Part model, mm, in its own coordinate system. Give positions to 0.01 mm unless a question says otherwise; leave off trailing zeros. Order: outer loops, then holes, each group sorted by start corner. A loop starts at its lowest first (then second) coordinate and runs counter-clockwise, first axis right, second up. Notation, with made-up numbers: (54.5, 38.25) -> (113.5, 38.25) arc R7 cw to (113.5, 49.25) -> close; hole circle Ø2 at (-16.5, 8). An arc over 180 degrees is marked (long way). Write item = value, one per line. Start each with the question number.
(1) Probe line 1 along X through (y, z) = (7.75, 940.5); line 2 along Z through (x, y) = (-110.5, 10.75); line 3 along X through (y, z) = (1.5, 679). List the from-to ranges inside material, lowest first. Write a range as from..to.
(2) Saw through at B-B, the plane y = 10. List the corners of the cut face in (x, z).
(3) Flat gauge pins, fed straight in: pin 1 (10.5 mm diameter, centred on y = 9.5, z = 1421, fed in from +X); pin 2 (8 mm diameter, centred on y = 8.5, z = 2045, fed in from +X); pin 3 (5 mm diameter, centred on x = -36.5, y = 9.5, fed in from -Z). Where does each tip first touch, or does it go through?
(4) Saw through at A-A, the plane z = 985.5. List the corners of the cut face in (x, y).
from build123d import *

# Parameters (mm, degrees)
F0_W     = 266.7
F0_H     = 9.525
F1_DEPTH = 2286
F2_DEPTH = 25.4
F3_W     = 266.7
F3_H     = 9.525
F4_DEPTH = 25.4


with BuildPart() as f1:
    # F0 (on Top) → F1 (new body)
    with BuildSketch(Plane.XY):
        with Locations((11.780921, 11.16089)):
            Rectangle(F0_W, F0_H)
        Polygon((-131.094079, 6.39839), (-140.619079, -3.12661), (164.180921, -3.12661), (154.655921, 6.39839), (145.130921, 6.39839), (-121.569079, 6.39839), align=None)
    extrude(amount=F1_DEPTH)

    # F0 (on Top) → F2 (cut)
    with BuildSketch(Plane.XY):
        with Locations((11.780921, 11.16089)):
            Rectangle(F0_W, F0_H)
    extrude(amount=F2_DEPTH, mode=Mode.SUBTRACT)

    # F3 (on face) → F4 (cut)
    with BuildSketch(Plane.XY.offset(2286)):
        with Locations((11.780921, 11.16089)):
            Rectangle(F3_W, F3_H)
    extrude(amount=-F4_DEPTH, mode=Mode.SUBTRACT)


solid = f1.part
Results list:
q1.line_1 = -121.57..145.13
q1.line_2 = 25.4..2260.6
q1.line_3 = -135.99..159.55
q2.outline = (-121.57, 25.4) -> (145.13, 25.4) -> (145.13, 2260.6) -> (-121.57, 2260.6) -> close
q3.pin_1 = 156.8
q3.pin_2 = 156.55
q3.pin_3 = 25.4
q4.outline = (-140.62, -3.13) -> (164.18, -3.13) -> (154.66, 6.4) -> (145.13, 6.4) -> (145.13, 15.92) -> (-121.57, 15.92) -> (-121.57, 6.4) -> (-131.09, 6.4) -> close
